Design review of the part built by this model. Coordinates are the model's own, in mm. A direction names the side the tool comes from. Round coordinates to 2 decimals unless told otherwise and drop trailing zeros. Order: outer loops, then holes, each group sorted by start corner. A loop starts at its lowest first (then second) coordinate and runs counter-clockwise, first axis right, second up.
from build123d import *

# Parameters (mm, degrees)
F1_DEPTH = 157.48
F2_R     = 3.175
F3_DEPTH = 438.151


with BuildPart() as f1:
    # F0 (on Front) → F1 (new body)
    with BuildSketch(Plane.XZ):
        with BuildLine():
            Line((-103.561188, -56.931033), (-103.561188, -63.281033))
            Line((-103.561188, -63.281033), (201.238812, -63.281033))
            Line((201.238812, -63.281033), (201.238812, -56.931033))
            Line((201.238812, -56.931033), (32.963812, -56.931033))
            ThreePointArc((32.963812, -56.931033), (30.718748, -56.001097), (29.788812, -53.756033))
            Line((29.788812, -53.756033), (29.788812, 349.468967))
            Line((29.788812, 349.468967), (23.438812, 349.468967))
            Line((23.438812, 349.468967), (23.438812, -53.756033))
            ThreePointArc((23.438812, -53.756033), (22.508876, -56.001097), (20.263812, -56.931033))
            Line((20.263812, -56.931033), (-103.561188, -56.931033))
        make_face()
        with BuildLine():
            Line((-408.361188, -63.281033), (-103.561188, -63.281033))
            Line((-103.561188, -63.281033), (-103.561188, -56.931033))
            Line((-103.561188, -56.931033), (-227.386188, -56.931033))
            ThreePointArc((-227.386188, -56.931033), (-229.631252, -56.001097), (-230.561188, -53.756033))
            Line((-230.561188, -53.756033), (-230.561188, 349.468967))
            Line((-230.561188, 349.468967), (-236.911188, 349.468967))
            Line((-236.911188, 349.468967), (-236.911188, -53.756033))
            ThreePointArc((-236.911188, -53.756033), (-237.841124, -56.001097), (-240.086188, -56.931033))
            Line((-240.086188, -56.931033), (-408.361188, -56.931033))
            Line((-408.361188, -56.931033), (-408.361188, -63.281033))
        make_face()
    extrude(amount=F1_DEPTH)

    # F2 (on face) → F3 (cut, through all)
    with BuildSketch(Plane(origin=(-236.911188, 0, 0), x_dir=(0, -1, 0), z_dir=(-1, 0, 0))):
        with Locations((40.64, 273.268967)):
            Circle(F2_R)
        with Locations((40.64, 197.068967)):
            Circle(F2_R)
        with Locations((40.64, 120.868967)):
            Circle(F2_R)
        with Locations((40.64, 44.668967)):
            Circle(F2_R)
        with Locations((116.84, 44.668967)):
            Circle(F2_R)
        with Locations((116.84, 120.868967)):
            Circle(F2_R)
        with Locations((116.84, 197.068967)):
            Circle(F2_R)
        with Locations((116.84, 273.268967)):
            Circle(F2_R)
    extrude(amount=-F3_DEPTH, mode=Mode.SUBTRACT)


solid = f1.part
1) Clearance check with flat-ended pins moving along their axes: P1, Ø2, axis at x = 117, y = -24.5, coming from the +Z side; P2, Ø10, axis at y = -116.84, z = 197.07, coming from the -X side; P3, Ø10, axis at y = -40.64, z = 273.27, coming from the +X side. State where each tip first meets the part, or that it passes through.
Results:
P1: stops at z = -56.93
P2: stops at x = -236.91
P3: stops at x = 29.79
2) To check wall thickness, follow line 1 along Z through (x, y) = (27, -116.84); line 2 along Z through (x, y) = (27, -116); line 3 along X through (y, z) = (-27, 264). State the ranges of each line that lie inside material, in increasing order.
Results:
line 1: z = -63.28 to 41.49, 47.84 to 117.69, 124.04 to 193.89, 200.24 to 270.09, 276.44 to 349.47
line 2: z = -63.28 to 41.61, 47.73 to 117.81, 123.93 to 194.01, 200.13 to 270.21, 276.33 to 349.47
line 3: x = -236.91 to -230.56, 23.44 to 29.79
3) The part is to be moulded in two halves that separate along X. For faces 5 (the face through (29.789, -78, 145)), 6 (the face through (-323, -78, -56.931)), 7 (the face through (-102, -78, -56.931)), 8 (the face through (23.439, -78, 151)), say which applies: released by +X, released by -X, zero draft, split by the parting line, or undercut.
Results:
face 5: released by +X
face 6: zero draft
face 7: undercut
face 8: undercut
4) For faces 1 (the face through (118, -78, -56.931)), 2 (the face through (-230.561, -78, 145)), 3 (the face through (-236.911, -78, 151)), 4 (the face through (-108, -78, -63.281)), list the 3-axis set-ups (+Z, -Z, +X, -X, +Y, -Y) from which the entire face can be reached by the end or side of a thin tool; tool diameter is ignored.
Results:
face 1: +Z, +X, +Y, -Y
face 2: +Z, +Y, -Y
face 3: +Z, -X, +Y, -Y
face 4: -Z, +X, -X, +Y, -Y
5) Take a section at C-C on x = -254.5. Give the boundary of the cut face in (y, z), plus the area to 4 significant figures.
Results:
outline: (-157.48, -63.28) - (0, -63.28) - (0, -56.93) - (-157.48, -56.93) - close
area: 1,000 mm2
6) Take a section at A-A on z = 234. Give the boundary of the cut face in (x, y).
Results:
outline: (-236.91, -157.48) - (-230.56, -157.48) - (-230.56, 0) - (-236.91, 0) - close; (23.44, -157.48) - (29.79, -157.48) - (29.79, 0) - (23.44, 0) - close
7) Take a section at B-B on y = -79. Give the boundary of the cut face in (x, z) (3 decimals), plus the area to 3 significant figures.
Results:
outline: (-408.361, -63.281) - (201.239, -63.281) - (201.239, -56.931) - (32.964, -56.931) arc R3.175 cw to (29.789, -53.756) - (29.789, 349.469) - (23.439, 349.469) - (23.439, -53.756) arc R3.175 cw to (20.264, -56.931) - (-227.386, -56.931) arc R3.175 cw to (-230.561, -53.756) - (-230.561, 349.469) - (-236.911, 349.469) - (-236.911, -53.756) arc R3.175 cw to (-240.086, -56.931) - (-408.361, -56.931) - close
area: 9,040 mm2
